CAD build for the part. Positions are in the model's coordinates, mm. A direction names the side the tool comes from. Coordinates: 2 decimals unless noted, no trailing zeros. Order: outer loops, then holes, each group sorted by start corner. A loop starts at its lowest first (then second) coordinate and runs counter-clockwise, first axis right, second up. Notation, with made-up numbers: M -3.75,74 L 8.25,74 A17 cw 8.25,107 Z; hole C 73,60 d9. An arc over 180 degrees is marked long. One line per item, written item: value.
from build123d import *

# Parameters (mm, degrees)
BOSS_EXTRUDE1_DEPTH = 10
CUT_EXTRUDE1_REACH  = 24.377
SKETCH2_R           = 1.7
FILLET1_R           = 1


with BuildPart() as part:
    # Sketch1 → Boss-Extrude1 (new body)
    with BuildSketch(Plane(origin=(0, 0, 0), x_dir=(1, 0, 0), z_dir=(0, 1, 0))):
        with BuildLine():
            Line((13.75, 3.269174208), (13.75, 16.887488657))
            Line((13.75, 16.887488657), (11.25, 16.887488657))
            Line((11.25, 16.887488657), (11.25, 5.910795209))
            ThreePointArc((11.25, 5.910795209), (15, -7), (18.75, 5.910795209))
            Line((18.75, 5.910795209), (18.75, 16.887488657))
            Line((18.75, 16.887488657), (16.25, 16.887488657))
            Line((16.25, 16.887488657), (16.25, 3.269174208))
            ThreePointArc((16.25, 3.269174208), (15, -3.5), (13.75, 3.269174208))
        make_face()
    extrude(amount=BOSS_EXTRUDE1_DEPTH)

    # Cut-Extrude1: up to this face of the body (flat: up to its plane)
    cut_extrude1_end = Plane(part.part.faces().sort_by_distance((11.25, 5, -11.399141933))[0])
    # Sketch2 → Cut-Extrude1 (cut, up to the picked face)
    with BuildSketch(Plane(origin=(18.75, 0, 0), x_dir=(0, 0, -1), z_dir=(1, 0, 0)), mode=Mode.PRIVATE) as cut_extrude1_sk1:
        with Locations((11.399141933, 5)):
            Circle(SKETCH2_R)
    cut_extrude1_tool1 = split(extrude(cut_extrude1_sk1.sketch, amount=-CUT_EXTRUDE1_REACH, mode=Mode.PRIVATE), bisect_by=cut_extrude1_end, keep=Keep.BOTH, mode=Mode.PRIVATE)
    add(cut_extrude1_tool1.solids().sort_by(Axis((18.75, 5, -11.399142), (-1, 0, 0)))[0], mode=Mode.SUBTRACT)

    # Fillet1
    fillet1_edges = [part.edges().sort_by_distance(p)[0] for p in [
        (15, 10, 3.5),
    ]]
    fillet(fillet1_edges, radius=FILLET1_R)


solid = part.part
Q1. Slice it at B-B (y = 5). List the corners of the cut face in (x, z).
Recorded:
outline: M 11.25,-16.89 L 13.75,-16.89 L 13.75,-13.1 L 11.25,-13.1 Z; M 11.25,-9.7 L 13.75,-9.7 L 13.75,-3.27 A3.5 cw long 16.25,-3.27 L 16.25,-9.7 L 18.75,-9.7 L 18.75,-5.91 A7 ccw long 11.25,-5.91 Z; M 16.25,-16.89 L 18.75,-16.89 L 18.75,-13.1 L 16.25,-13.1 Z
Q2. Which spindle directions (+Z, -Z, +X, -X, +Y, -Y) get a long thin tool onto all of the face, cutting with end or side? Do faces 1 (the face through (11.25, 4, -13)), 2 (the face through (13.75, 5, -8)), 3 (the face through (16.5, 0, -5.1)), 4 (the face through (18.75, 3, -11)). Say none if no direction does.
Recorded:
face 1: -Z, -X, +Y, -Y
face 2: -Z, +Y, -Y
face 3: +Z, -Z, +X, -X, -Y
face 4: -Z, +X, +Y, -Y
Q3. Pin check, flat tips, straight feed: pin 1 Ø5 at (y, z) = (5, -11.5) entering from -X; pin 2 Ø3 at (y, z) = (3, -10.5) entering from +X; pin 3 Ø1 at (y, z) = (5.5, -3) entering from -X. Stop position of each tip, or through.
Recorded:
pin 1: stops at x = 11.25
pin 2: stops at x = 18.75
pin 3: stops at x = 8.46
Q4. Slice it at C-C (z = -11.75). List the corners of the cut face in (x, y), plus the area to 3 significant figures.
Recorded:
outline: M 11.25,0 L 13.75,0 L 13.75,3.34 L 11.25,3.34 Z; M 11.25,6.66 L 13.75,6.66 L 13.75,10 L 11.25,10 Z; M 16.25,0 L 18.75,0 L 18.75,3.34 L 16.25,3.34 Z; M 16.25,6.66 L 18.75,6.66 L 18.75,10 L 16.25,10 Z
area: 33.4 mm^2
Q5. Drill centre lines: line 1 along X through (y, z) = (8.5, -12.75); line 2 along Z through (x, y) = (13.5, 6.25); line 3 along X through (y, z) = (7.75, -4). Where is each one in solid material? Low to high.
Recorded:
line 1: x = 11.25 to 13.75, 16.25 to 18.75
line 2: z = -16.89 to -12.55, -10.25 to -3.16, 3.16 to 6.84
line 3: x = 9.26 to 13.75, 16.25 to 20.74
Q6. Mould opens along Z. For faces 5 (the face through (15.1, 4.4, 3.5)), 6 (the face through (15, 5, 7)), 7 (the face through (13, 10, -5)), 8 (the face through (13, 5, -16.887)) say: released by +Z, released by -Z, zero draft, split by the parting line, or undercut.
Recorded:
face 5: undercut
face 6: split by the parting line
face 7: zero draft
face 8: released by -Z
Q7. Slice it at D-D (y = 8). List the corners of the cut face in (x, z).
Recorded:
outline: M 11.25,-16.89 L 13.75,-16.89 L 13.75,-3.27 A3.5 cw long 16.25,-3.27 L 16.25,-16.89 L 18.75,-16.89 L 18.75,-5.91 A7 ccw long 11.25,-5.91 Z
Q8. Slice it at A-A (z = -15.25). List the corners of the cut face in (x, y).
Recorded:
outline: M 11.25,0 L 13.75,0 L 13.75,10 L 11.25,10 Z; M 16.25,0 L 18.75,0 L 18.75,10 L 16.25,10 Z
